Can you work these out from the model? Positions are in its coordinate system, mm. Round coordinates to 2 decimals unless told otherwise and drop trailing zeros. Write each loop counter-clockwise with the first axis right and the second up, starting at its lowest first coordinate (ties: lowest second). Pieces come first, ordered by that corner, then holes. Notation, with made-up numbers: (21, 63) -> (29, 63) arc R12 ccw to (29, 76) -> close; hole circle Ø7 at (-39, -30). An arc over 180 degrees is marked (long way). Use CSV: the item, a comma, the result in double quotes.
```python
from build123d import *

# Parameters (mm, degrees)
SKETCH_1_W          = 10
SKETCH_1_H          = 10
SKETCH_1_W_2        = 8
SKETCH_1_H_2        = 8
EXTRUDE_1_DEPTH     = 175
SKETCH_2_R          = 2.15
CUT_EXTRUDE_1_DEPTH = 176.356779168
SKETCH_3_R          = 1.6
SKETCH_3_R_2        = 2.15
CUT_EXTRUDE_2_DEPTH = 176.356779168
SKETCH_4_R          = 4
CUT_EXTRUDE_3_DEPTH = 9


with BuildPart() as part:
    # ｽｹｯﾁ1 → 押し出し-薄板1 (new body)
    with BuildSketch(Plane.XY):
        Rectangle(SKETCH_1_W, SKETCH_1_H)
        Rectangle(SKETCH_1_W_2, SKETCH_1_H_2, mode=Mode.SUBTRACT)
    extrude(amount=EXTRUDE_1_DEPTH)

    # ｽｹｯﾁ2 → ｶｯﾄ - 押し出し1 (cut, through all)
    with BuildSketch(Plane(origin=(5, 0, 0), x_dir=(0, 0, -1), z_dir=(1, 0, 0))):
        with Locations(Location((-170, 0, 0), (0, 0, 90))):
            Circle(SKETCH_2_R)
        with Locations(Location((-5, 0, 0), (0, 0, 270))):
            Circle(SKETCH_2_R)
    extrude(amount=-CUT_EXTRUDE_1_DEPTH, mode=Mode.SUBTRACT)

    # ｽｹｯﾁ3 → ｶｯﾄ - 押し出し2 (cut, through all)
    with BuildSketch(Plane(origin=(0, 5, 0), x_dir=(1, 0, 0), z_dir=(0, 1, 0))):
        with Locations(Location((0, -76.5, 0), (0, 0, 180))):
            Circle(SKETCH_3_R)
        with Locations(Location((0, -56.5, 0), (0, 0, 180))):
            Circle(SKETCH_3_R)
        with Locations(Location((0, -87.5, 0), (0, 0, 180))):
            Circle(SKETCH_3_R_2)
    extrude(amount=-CUT_EXTRUDE_2_DEPTH, mode=Mode.SUBTRACT)

    # ｽｹｯﾁ4 → ｶｯﾄ - 押し出し3 (cut)
    with BuildSketch(Plane.XZ.offset(5)):
        with Locations((0, 87.5)):
            Circle(SKETCH_4_R)
    extrude(amount=-CUT_EXTRUDE_3_DEPTH, mode=Mode.SUBTRACT)


solid = part.part
```
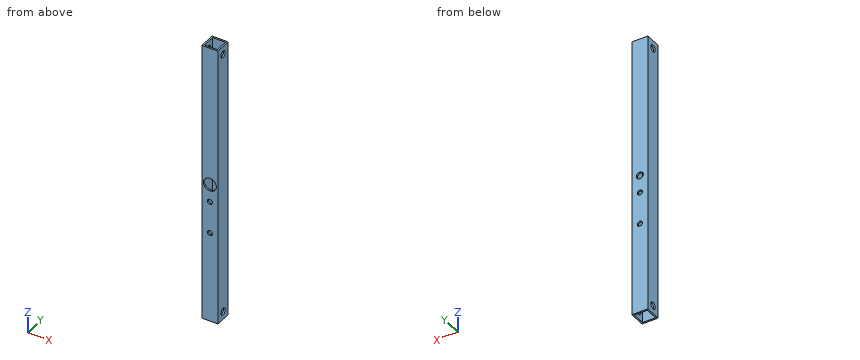
Q1. Suppose I cut it at C-C (x = 0). Count the separate pieces of the cut face and the enclosed holes in it, and give its area (3 significant figures).
Resolved:
separate pieces,"8"
enclosed holes,"0"
area,"325 mm^2"
Q2. Suppose I cut it at B-B (z = 20). Write out the boundary of the cut face in (x, y).
Resolved:
outline,"(-5, -5) -> (5, -5) -> (5, 5) -> (-5, 5) -> close; hole (-4, -4) -> (4, -4) -> (4, 4) -> (-4, 4) -> close"
Q3. Will this pin go through, and if not, where does the flat tip stop? P1, Ø3.5, axis at x = 0, z = 87.5, coming from the +Y side.
Resolved:
P1,"passes through"
Q4. Suppose I cut it at A-A (y = 0). Write out the boundary of the cut face in (x, z), and give its area (3 significant figures).
Resolved:
outline,"(-5, 0) -> (-4, 0) -> (-4, 2.85) -> (-5, 2.85) -> close; (-5, 7.15) -> (-4, 7.15) -> (-4, 167.85) -> (-5, 167.85) -> close; (-5, 172.15) -> (-4, 172.15) -> (-4, 175) -> (-5, 175) -> close; (4, 0) -> (5, 0) -> (5, 2.85) -> (4, 2.85) -> close; (4, 7.15) -> (5, 7.15) -> (5, 167.85) -> (4, 167.85) -> close; (4, 172.15) -> (5, 172.15) -> (5, 175) -> (4, 175) -> close"
area,"333 mm^2"
Q5. Please list where these lines run through material, in increasing order: probe 1 along Z at (x, y) = (-4.6, 0); probe 2 along Y at (x, z) = (1, 141.5).
Resolved:
probe 1,"z = 0 to 2.85, 7.15 to 167.85, 172.15 to 175"
probe 2,"y = -5 to -4, 4 to 5"
Q6. Suppose I cut it at D-D (z = 76.5). Write out the boundary of the cut face in (x, y), and give its area (3 significant figures).
Resolved:
outline,"(-5, -5) -> (-1.6, -5) -> (-1.6, -4) -> (-4, -4) -> (-4, 4) -> (-1.6, 4) -> (-1.6, 5) -> (-5, 5) -> close; (1.6, -5) -> (5, -5) -> (5, 5) -> (1.6, 5) -> (1.6, 4) -> (4, 4) -> (4, -4) -> (1.6, -4) -> close"
area,"29.6 mm^2"
